Can you work these out from the drawing? Everything is in mm from the part's minimum corner. A direction names the side the tool comes from. Coordinates: 2 decimals unless noted, no trailing zeros. Order: outer loops, then holes, each group sorted by start corner. A loop starts at its lowest first (then second) coordinate and runs counter-clockwise, first axis right, second up. Notation, with made-up numbers: M -11.5,73.25 L 8.5,73.25 A15 ccw 8.5,89.25 Z; hole C -19.5,67.25 d8. An arc over 180 degrees is marked long. Answer as a JSON object with one key per item and string values.
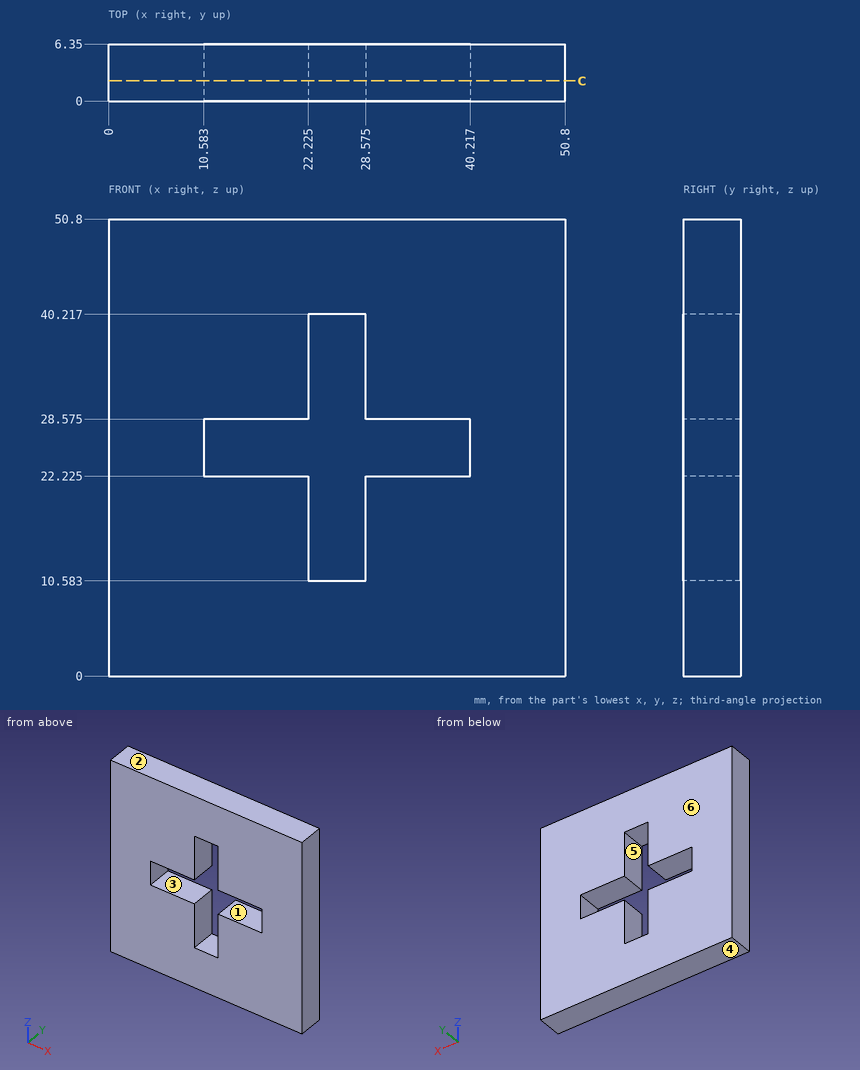
Item 1: I'm going to push a flat-ended pin straight in: pin 1 (1.9 mm diameter, centred on x = 34, y = 2.5, fed in from -Z). Where does the tip first touch, or does it pass through?
Answers follow:
{"pin 1": "stops at z = 0"}
Item 2: Which directions (+Z, -Z, +X, -X, +Y, -Y) give clear straight access to the entire face, cutting with the end or side of a thin tool? Please do the marked faces 1 and 2.
Answers follow:
{"face 1": "+Y, -Y", "face 2": "+Z, +X, -X, +Y, -Y"}
Item 3: I want a section at C-C, the plane y = 2.25. Write out the boundary of the cut face in (x, z) (1 decimal).
Answers follow:
{"outline": "M 0,0 L 50.8,0 L 50.8,50.8 L 0,50.8 Z; hole M 10.6,22.2 L 22.2,22.2 L 22.2,10.6 L 28.6,10.6 L 28.6,22.2 L 40.2,22.2 L 40.2,28.6 L 28.6,28.6 L 28.6,40.2 L 22.2,40.2 L 22.2,28.6 L 10.6,28.6 Z"}
Item 4: If we mould it in two halves opening along Z, with no side actions, what happens to the marked faces 3, 4, 5 and 6? For each: pulls with the +Z half, pulls with the -Z half, needs draft (parallel to the pull), parting line crosses it, or undercut.
Answers follow:
{"face 3": "undercut", "face 4": "pulls with the -Z half", "face 5": "undercut", "face 6": "needs draft"}
Item 5: Please list where these lines run through material, in increasing order: line 1 (Z direction, x = 26, y = 4.5); line 2 (X direction, y = 5.75, z = 18) (1 decimal).
Answers follow:
{"line 1": "z = 0 to 10.58, 40.22 to 50.8", "line 2": "x = 0 to 22.2, 28.6 to 50.8"}
